from build123d import *

# Parameters (mm, degrees)
BOSS_EXTRUDE1_DEPTH = 50
SKETCH4_W           = 40
SKETCH4_H           = 47.735026919
CUT_EXTRUDE1_DEPTH  = 1340.48308574


with BuildPart() as part:
    # Sketch3 → Boss-Extrude1 (new body)
    with BuildSketch(Plane.XY):
        Polygon((0, 0), (-1157.735026919, 0), (-1128.867513459, -50), (-28.867513459, -50), align=None)
    extrude(amount=BOSS_EXTRUDE1_DEPTH)

    # Sketch4 → Cut-Extrude1 (cut, through all, along a direction that is not the sketch's normal)
    with BuildSketch(Plane(origin=(0, 0, 0), x_dir=(0, 0, -1), z_dir=(0.8660254037844366, -0.5000000000000037, 0))):
        with Locations((-25, -28.86751346)):
            Rectangle(SKETCH4_W, SKETCH4_H)
    extrude(amount=-CUT_EXTRUDE1_DEPTH, dir=(1, 0, 0), mode=Mode.SUBTRACT)


solid = part.part
Can you work these out from the model? Positions are in its coordinate system, mm. A direction names the side the tool comes from. Coordinates: 2 decimals unless noted, no trailing zeros. Order: outer loops, then holes, each group sorted by start corner. A loop starts at its lowest first (then second) coordinate and runs counter-clockwise, first axis right, second up. Notation, with made-up numbers: (37.25, 71) - (56.25, 71) arc R21 ccw to (56.25, 89) - close; hole circle Ø6 at (73, 67.25). An arc over 180 degrees is marked (long way). Answer as a JSON object with one key per item and string values. Group by question number.
Q1. On a 3-axis mill with a long thin cutter (end or side, diameter ignored), from which of +Z, -Z, +X, -X, +Y, -Y can I reach the whole of each face in a straight line? I mean faces 1 (the face through (-571, 0, 25)), 2 (the face through (-571, -45.67, 25)). Say none if no direction works.
Q2. Will this pin go through, and if not, where does the flat tip stop? P1, Ø8, axis at y = -15, z = 10.5, coming from the -X side.
Q3. Imagine slicing it at A-A (x = -316.5). Please give me the cut outline in (y, z), and give its area (3 significant figures).
Q4. Imagine slicing it at C-C (z = 12.5). Please give me the cut outline in (x, y), and give its area (3 significant figures).
Q5. Imagine slicing it at B-B (y = -31). Please give me the cut outline in (x, z), and give its area (3 significant figures).
Q6. We'd pull the mould along Y, two halves only. Please class faces 3 (the face through (-587, -25, 0)), 4 (the face through (-571, -4.33, 25)), 5 (the face through (-14.636, -25.35, 46.872)): +Y half, -Y half, draft (parallel to the pull), parting line (faces both ways), or undercut.
Q7. I need wall thicknesses on line 1 (Z direction, x = -604.5, y = -13); line 2 (Y direction, x = -239, z = 10); line 3 (X direction, y = -4, z = 5). Which ranges of each line are inside material? Lowest first, please. Write a range as from..to.
Determined:
{
 "1": {"face 1": "+Z, -Z, +X, -X, +Y", "face 2": "+X, -X"},
 "2": {"P1": "passes through"},
 "3": {"outline": "(-50, 0) - (0, 0) - (0, 50) - (-50, 50) - close; hole (-45.67, 5) - (-4.33, 5) - (-4.33, 45) - (-45.67, 45) - close", "area": "846 mm2"},
 "4": {"outline": "(-1157.74, 0) - (-1155.24, -4.33) - (-2.5, -4.33) - (0, 0) - close; (-1131.37, -45.67) - (-1128.87, -50) - (-28.87, -50) - (-26.37, -45.67) - close", "area": "9,780 mm2"},
 "5": {"outline": "(-1139.84, 0) - (-17.9, 0) - (-17.9, 5) - (-1139.84, 5) - close; (-1139.84, 45) - (-17.9, 45) - (-17.9, 50) - (-1139.84, 50) - close", "area": "11,200 mm2"},
 "6": {"face 3": "draft", "face 4": "undercut", "face 5": "-Y half"},
 "7": {"line 1": "z = 0..5, 45..50", "line 2": "y = -50..-45.67, -4.33..0", "line 3": "x = -1155.43..-2.31"}
}
